```python
from build123d import *

# Parameters (mm, degrees)
SKETCH_1_W                       = 400
SKETCH_1_H                       = 135
SKETCH_1_R                       = 3
SM_BASE_FLANGE_1_DEPTH           = 0.7
SM_EDGE_FLANGE_1_STRIP_W         = 3.2
SM_EDGE_FLANGE_1_STRIP_H         = 0.7
SM_EDGE_FLANGE_1_STRIP_CUT_DEPTH = 400
SM_EDGE_FLANGE_1_DEPTH           = 400
OTHER_START                      = -200
OTHER_1_DEPTH                    = 400
OTHER_1_2_DEPTH                  = 400


# Read off the part's stored shape, not the designer's step: 褶边1
# Sheet-metal steps are written as plain solids
with BuildPart() as part:
    # Sketch 1 → 基体-法兰1 (new body)
    with BuildSketch(Plane(origin=(0, 0, 0), x_dir=(1, 0, 0), z_dir=(0, 1, 0))):
        Rectangle(SKETCH_1_W, SKETCH_1_H)
        with Locations(Location((-194.5, -60.5, 0), (0, 0, 270))):
            Circle(SKETCH_1_R, mode=Mode.SUBTRACT)
        with Locations(Location((-194.5, -10.5, 0), (0, 0, 270))):
            Circle(SKETCH_1_R, mode=Mode.SUBTRACT)
        with Locations(Location((-194.5, -0.5, 0), (0, 0, 270))):
            Circle(SKETCH_1_R, mode=Mode.SUBTRACT)
        with Locations(Location((-194.5, 49.5, 0), (0, 0, 270))):
            Circle(SKETCH_1_R, mode=Mode.SUBTRACT)
        with Locations(Location((0, -10.5, 0), (0, 0, 270))):
            Circle(SKETCH_1_R, mode=Mode.SUBTRACT)
        with Locations(Location((0, -0.5, 0), (0, 0, 270))):
            Circle(SKETCH_1_R, mode=Mode.SUBTRACT)
        with Locations(Location((194.5, -60.5, 0), (0, 0, 90))):
            Circle(SKETCH_1_R, mode=Mode.SUBTRACT)
        with Locations(Location((194.5, -10.5, 0), (0, 0, 90))):
            Circle(SKETCH_1_R, mode=Mode.SUBTRACT)
        with Locations(Location((194.5, -0.5, 0), (0, 0, 90))):
            Circle(SKETCH_1_R, mode=Mode.SUBTRACT)
        with Locations(Location((194.5, 49.5, 0), (0, 0, 90))):
            Circle(SKETCH_1_R, mode=Mode.SUBTRACT)
    extrude(amount=-SM_BASE_FLANGE_1_DEPTH)

    # 边线-法兰1 strip (across the edge) → 边线-法兰1 strip cut (cut)
    with BuildSketch(Plane(origin=(-200, -0.7, -67.5), x_dir=(0, 0, 1), z_dir=(1, 0, 0))):
        with Locations((-0.7, -0.35)):
            Rectangle(SM_EDGE_FLANGE_1_STRIP_W, SM_EDGE_FLANGE_1_STRIP_H)
    extrude(amount=SM_EDGE_FLANGE_1_STRIP_CUT_DEPTH, mode=Mode.SUBTRACT)

    # 边线-法兰1 section (across the edge) → 边线-法兰1 (add)
    with BuildSketch(Plane(origin=(-200, -0.7, -67.5), x_dir=(0, 0, 1), z_dir=(1, 0, 0))):
        with BuildLine():
            Line((0, 0.2), (0, 5.3))
            Line((0, 5.3), (0.7, 5.3))
            Line((0.7, 5.3), (0.7, 0.2))
            ThreePointArc((0.7, 0.2), (0.758578644, 0.058578644), (0.9, 0))
            Line((0.9, 0), (0.9, -0.7))
            ThreePointArc((0.9, -0.7), (0.263603897, -0.436396103), (0, 0.2))
        make_face()
    extrude(amount=SM_EDGE_FLANGE_1_DEPTH)

    # Other 1 outline → Other 1 (cut)
    with BuildSketch(Plane.YZ.offset(OTHER_START)):
        with BuildLine():
            Line((-6, -67.5), (-5.890871211, -67.5))
            ThreePointArc((-5.890871211, -67.5), (-5.44807407, -66.990049506), (-4.8, -66.8))
            Line((-4.8, -66.8), (-6, -66.8))
            Line((-6, -66.8), (-6, -67.5))
        make_face()
    extrude(amount=OTHER_1_DEPTH, mode=Mode.SUBTRACT)

    # Other 1 2 outline → Other 1 2 (add)
    with BuildSketch(Plane.YZ.offset(OTHER_START)):
        with BuildLine():
            Line((-1, -69.2), (-1, -68.5))
            Line((-1, -68.5), (-4.8, -68.5))
            ThreePointArc((-4.8, -68.5), (-5.3, -68), (-4.8, -67.5))
            Line((-4.8, -67.5), (-5.890871211, -67.5))
            ThreePointArc((-5.890871211, -67.5), (-5.809950494, -68.64807407), (-4.8, -69.2))
            Line((-4.8, -69.2), (-1, -69.2))
        make_face()
    extrude(amount=OTHER_1_2_DEPTH)


solid = part.part
```
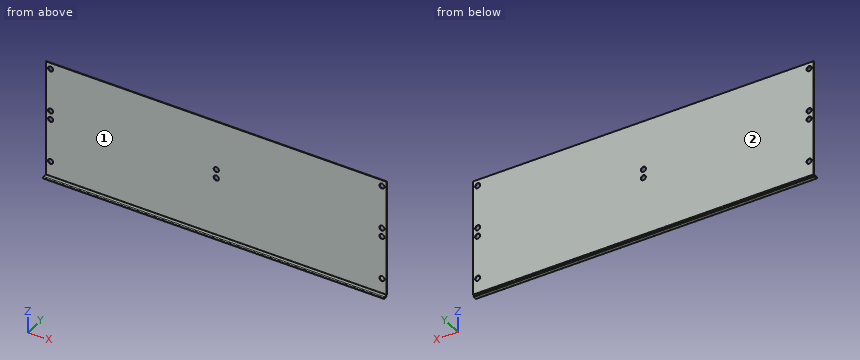
Input: part model. Units: mm. Frame: model coordinates. Face numbers are marked on the shaded views. A direction names the side the tool comes from. Give positions to 0.01 mm unless a question says otherwise; leave off trailing zeros. Order: outer loops, then holes, each group sorted by start corner. A loop starts at its lowest first (then second) coordinate and runs counter-clockwise, first axis right, second up. Notation, with made-up numbers: (40.5, 5) - (74.5, 5) arc R33 cw to (74.5, 41) - close; hole circle Ø6 at (10.5, 42). An arc over 180 degrees is marked (long way). One line per item, written item: value.
1. Cut plane A-A, the plane y = -3.15. Output: boundary loops of the cut face in (x, z), and give its area (3 significant figures).
Determined:
outline: (-200, -69.2) - (200, -69.2) - (200, -68.5) - (-200, -68.5) - close; (-200, -67.5) - (200, -67.5) - (200, -66.8) - (-200, -66.8) - close
area: 560 mm2
2. Cut plane C-C, the plane z = 22. Output: boundary loops of the cut face in (x, y).
Determined:
outline: (-200, -0.7) - (200, -0.7) - (200, 0) - (-200, 0) - close
3. Line query: probe 1 along X at (y, z) = (-0.25, 0.5); probe 2 along X at (y, z) = (-0.5, 60.5); probe 3 along Z at (x, y) = (-85.5, -3.15). Output: solid intervals per line, ascending.
Determined:
probe 1: -200 to -197.5, -191.5 to -3, 3 to 191.5, 197.5 to 200
probe 2: -200 to -197.5, -191.5 to 191.5, 197.5 to 200
probe 3: -69.2 to -68.5, -67.5 to -66.8
4. Reachability of the marked faces 1 and 2 from +Z, -Z, +X, -X, +Y, -Y: full face, straight path, thin tool, end or side. Return the list, or none.
Determined:
face 1: +Z, +X, -X, -Y
face 2: +Z, -Z, +X, -X, +Y
5. Cut plane B-B, the plane x = 141.5. Output: boundary loops of the cut face in (y, z), and give its area (3 significant figures).
Determined:
outline: (-4.8, -69.2) - (-1, -69.2) - (-1, -68.5) - (-4.8, -68.5) arc R0.5 cw to (-4.8, -67.5) - (-0.9, -67.5) arc R0.9 ccw to (0, -66.6) - (0, 67.5) - (-0.7, 67.5) - (-0.7, -66.6) arc R0.2 cw to (-0.9, -66.8) - (-4.8, -66.8) arc R1.2 ccw to start
area: 102 mm2
6. Pin query (flat end, axial travel): pin 1 Ø1 at (x, z) = (-101, -46.5) entering from -Y; pin 2 Ø2 at (x, y) = (-90.5, -2) entering from +Z. Return the tip coordinate at first contact, or that it passes through.
Determined:
pin 1: y = -0.7
pin 2: z = -66.8
